```python
from build123d import *

# Parameters (mm, degrees)
F0_W     = 80
F0_H     = 26
F0_R     = 1.85
F1_DEPTH = 25
F3_R     = 3.25
F3_R_2   = 1.85
F4_DEPTH = 21
F5_DEPTH = 100


with BuildPart() as f1:
    # F0 (on Top) → F1 (new body)
    with BuildSketch(Plane.XY):
        Rectangle(F0_W, F0_H)
        with Locations((-32, -8)):
            Circle(F0_R, mode=Mode.SUBTRACT)
        with Locations((0, -8)):
            Circle(F0_R, mode=Mode.SUBTRACT)
        with Locations((32, -8)):
            Circle(F0_R, mode=Mode.SUBTRACT)
        with Locations((-32, 8)):
            Circle(F0_R, mode=Mode.SUBTRACT)
        with Locations((0, 8)):
            Circle(F0_R, mode=Mode.SUBTRACT)
        with Locations((32, 8)):
            Circle(F0_R, mode=Mode.SUBTRACT)
    extrude(amount=F1_DEPTH)

    # F3 (on face) → F4 (cut)
    with BuildSketch(Plane.XY.offset(25)):
        with Locations((-32, -8)):
            Circle(F3_R)
        with Locations((-32, -8)):
            Circle(F3_R_2, mode=Mode.SUBTRACT)
        with Locations((-32, 8)):
            Circle(F3_R)
        with Locations((-32, 8)):
            Circle(F3_R_2, mode=Mode.SUBTRACT)
        with Locations((0, 8)):
            Circle(F3_R)
        with Locations((0, 8)):
            Circle(F3_R_2, mode=Mode.SUBTRACT)
        with Locations((0, -8)):
            Circle(F3_R)
        with Locations((0, -8)):
            Circle(F3_R_2, mode=Mode.SUBTRACT)
        with Locations((32, 8)):
            Circle(F3_R)
        with Locations((32, 8)):
            Circle(F3_R_2, mode=Mode.SUBTRACT)
        with Locations((32, -8)):
            Circle(F3_R)
        with Locations((32, -8)):
            Circle(F3_R_2, mode=Mode.SUBTRACT)
    extrude(amount=-F4_DEPTH, mode=Mode.SUBTRACT)

    # F2 (on face) → F5 (cut)
    with BuildSketch(Plane.YZ.offset(40)):
        with BuildLine():
            Line((-13, 25), (-13, 12))
            ThreePointArc((-13, 12), (0, 6), (13, 12))
            Line((13, 12), (13, 25))
            Line((13, 25), (-13, 25))
        make_face()
    extrude(amount=-F5_DEPTH, mode=Mode.SUBTRACT)


solid = f1.part
```
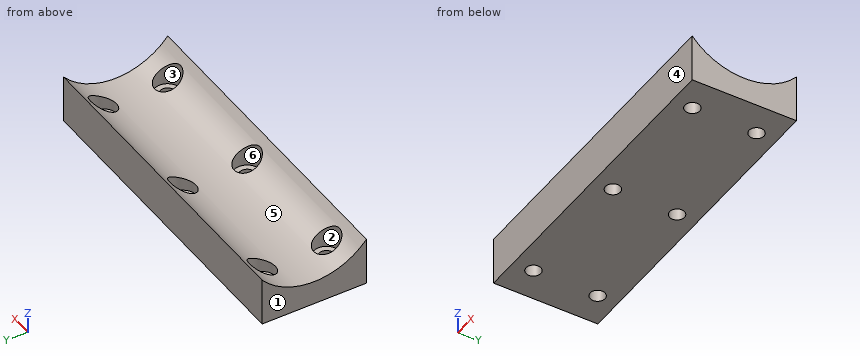
The model under review builds one solid part; all positions refer to its coordinate system, in mm. Face numbers are marked on the shaded views. A direction names the side the tool comes from. Round coordinates to 2 decimals unless told otherwise and drop trailing zeros. Write each loop counter-clockwise with the first axis right and the second up, starting at its lowest first coordinate (ties: lowest second). Pieces come first, ordered by that corner, then holes.
(1) Machinability: for the marked faces 5 and 6, which of the approach directions +Z, -Z, +X, -X, +Y, -Y give a long, thin tool a straight path to every point of the face, cutting with its end or side? Answer none if there is none.
(2) Insertion check: pin 1 (2 mm diameter, centred on x = -31, y = -7.5, fed in from +Z); pin 2 (8.5 mm diameter, centred on x = 32, y = 8, fed in from +Z); pin 3 (7 mm diameter, centred on x = 31.5, y = -8.5, fed in from +Z). Each pin has a flat end and moves straight along its axis. Give the tip position at first contact, or say it passes through.
(3) We need section B-B on x = 0. Give the boundary of the cut face in (y, z), and give its area (3 significant figures).
(4) We need section A-A on y = -8. Give the boundary of the cut face in (x, z), and give its area (3 significant figures).
(5) Wall thickness on L1, parallel to Y at x = -32, z = 2.35; L2, parallel to X at y = -8, z = 5.75; L3, parallel to X at y = 7.75, z = 0.5: over which ranges is each line inside the solid? List them lowest first.
(6) Mouldability with a two-part tool opening along X and no side actions: class the marked faces 1, 2, 3 and 4 as +X half, -X half, draft (parallel to the pull), parting line (faces both ways), or undercut.
(7) We need section C-C on y = -0.25. Give the boundary of the cut face in (x, z).
Findings below:
1. face 5: +Z, +X, -X
1. face 6: +Z
2. pin 1: stops at z = 4
2. pin 2: stops at z = 11.18
2. pin 3: stops at z = 10.92
3. outline: (-13, 0) - (-9.85, 0) - (-9.85, 4) - (-11.25, 4) - (-11.25, 10.23) arc R17.08 cw to (-13, 12) - close; (-6.15, 0) - (6.15, 0) - (6.15, 4) - (4.75, 4) - (4.75, 6.67) arc R17.08 cw to (-4.75, 6.67) - (-4.75, 4) - (-6.15, 4) - close; (9.85, 0) - (13, 0) - (13, 12) arc R17.08 cw to (11.25, 10.23) - (11.25, 4) - (9.85, 4) - close
3. area: 120 mm2
4. outline: (-40, 0) - (-33.85, 0) - (-33.85, 4) - (-35.25, 4) - (-35.25, 7.99) - (-40, 7.99) - close; (-30.15, 0) - (-1.85, 0) - (-1.85, 4) - (-3.25, 4) - (-3.25, 7.99) - (-28.75, 7.99) - (-28.75, 4) - (-30.15, 4) - close; (1.85, 0) - (30.15, 0) - (30.15, 4) - (28.75, 4) - (28.75, 7.99) - (3.25, 7.99) - (3.25, 4) - (1.85, 4) - close; (33.85, 0) - (40, 0) - (40, 7.99) - (35.25, 7.99) - (35.25, 4) - (33.85, 4) - close
4. area: 517 mm2
5. L1: y = -13 to -9.85, -6.15 to 6.15, 9.85 to 13
5. L2: x = -40 to -35.25, -28.75 to -3.25, 3.25 to 28.75, 35.25 to 40
5. L3: x = -40 to -33.83, -30.17 to -1.83, 1.83 to 30.17, 33.83 to 40
6. face 1: -X half
6. face 2: undercut
6. face 3: undercut
6. face 4: draft
7. outline: (-40, 0) - (40, 0) - (40, 6) - (-40, 6) - close
